Could you check a few things on this drawing? It's one solid part, dimensions in mm from its lowest x, y, z. Round coordinates to 2 decimals unless told otherwise and drop trailing zeros. Order: outer loops, then holes, each group sorted by start corner. A loop starts at its lowest first (then second) coordinate and runs counter-clockwise, first axis right, second up.
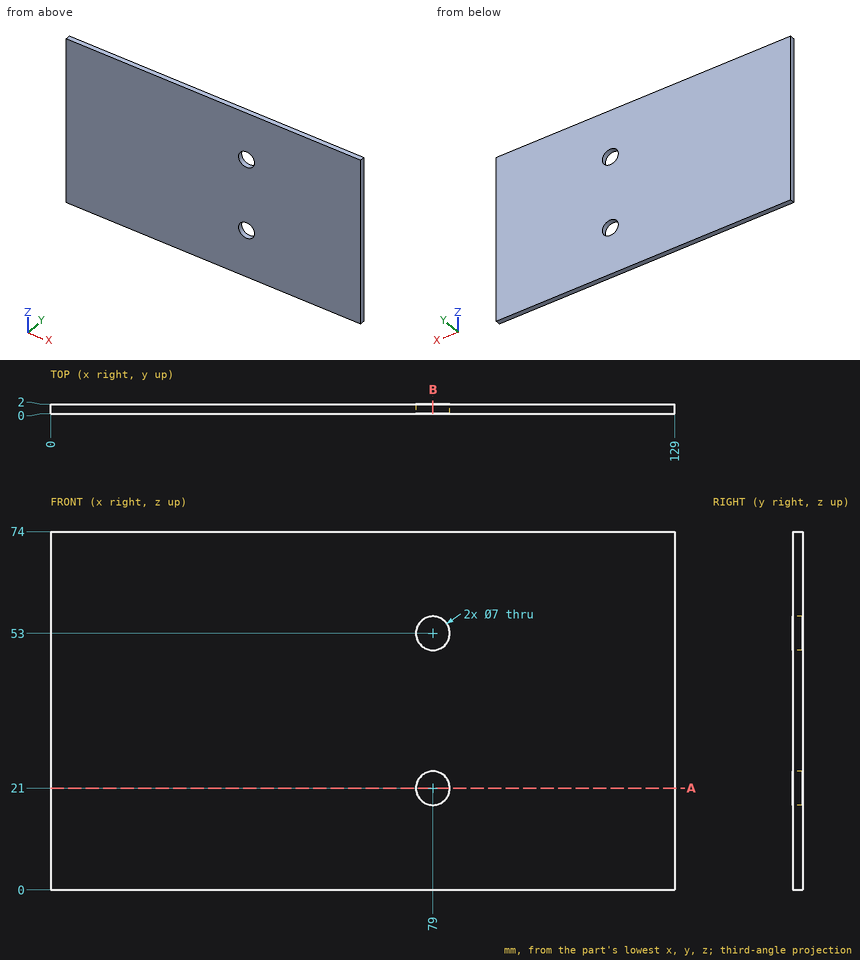
1) If we section it at B-B (x = 79): Write out the boundary of the cut face in (y, z), plus the area to 3 significant figures.
2) I need wall thicknesses on line 1 (Z direction, x = 79, y = 0.9); line 2 (X direction, y = 0.9, z = 22.5). Which ranges of each line are inside material? Lowest first, please.
3) If we section it at A-A (z = 21): Write out the boundary of the cut face in (x, y).
Solutions:
1. outline: (0, 0) - (2, 0) - (2, 17.5) - (0, 17.5) - close; (0, 24.5) - (2, 24.5) - (2, 49.5) - (0, 49.5) - close; (0, 56.5) - (2, 56.5) - (2, 74) - (0, 74) - close
1. area: 120 mm2
2. line 1: z = 0 to 17.5, 24.5 to 49.5, 56.5 to 74
2. line 2: x = 0 to 75.84, 82.16 to 129
3. outline: (0, 0) - (75.5, 0) - (75.5, 2) - (0, 2) - close; (82.5, 0) - (129, 0) - (129, 2) - (82.5, 2) - close
